```python
from build123d import *

# Parameters (mm, degrees)
F0_R     = 40.5
F1_DEPTH = 165
F2_W     = 77
F2_H     = 150
F3_DEPTH = 50.000001
F4_T     = -1.5
F5_R     = 40
F6_DEPTH = 165


with BuildPart() as f1:
    # F0 (on Top) → F1 (new body)
    with BuildSketch(Plane.XY):
        Circle(F0_R)
    extrude(amount=F1_DEPTH)

    # F2 (on Front) → F3 (cut)
    with BuildSketch(Plane.XZ):
        with Locations((0, 83.080945)):
            Rectangle(F2_W, F2_H)
    extrude(amount=F3_DEPTH, mode=Mode.SUBTRACT)

    # F4
    f4_openings = [f1.faces().sort_by_distance(p)[0] for p in [
        (0, 0, 165),
    ]]
    offset(amount=F4_T, openings=f4_openings)

    # F5 (on Top) → F6 (cut)
    with BuildSketch(Plane.XY):
        Circle(F5_R)
    extrude(amount=F6_DEPTH, mode=Mode.SUBTRACT)


solid = f1.part
```
Geometry check sheet. Reference: the model listing, model coordinates, mm. Coordinates: 2 decimals unless noted, no trailing zeros. Loops run counter-clockwise (first coordinate to the right, second up) from the corner with the lowest first, then second, coordinate; pieces in that order, holes last.
Item 1: Go/stop test with flat-tipped pins: pin 1 Ø6 at (x, z) = (-14, 104) entering from +Y; pin 2 Ø8 at (y, z) = (19, 128.5) entering from -X; pin 3 Ø9 at (x, y) = (-2.5, -32) entering from -Z; pin 4 Ø1 at (y, z) = (7.5, 21) entering from +X. Record where each tip stops, or that it passes through.
Item 2: Sectioned sample at D-D, the plane x = 25. Record the boundary of the cut face in (y, z), then the cut area to 3 significant figures.
Item 3: Sectioned sample at B-B, the plane x = 0. Record the boundary of the cut face in (y, z).
Item 4: Release check for a two-part mould opening along Z. For faces 1 (the face through (5.5, -39.9, 158.081)), 2 (the face through (-9.2, 39.2, 165)), 3 (the face through (-9.2, 39.2, 0)) record: released by +Z, released by -Z, zero draft, split by the parting line, or undercut.
Item 5: Sectioned sample at C-C, the plane y = -15.5. Record the boundary of the cut face in (x, z).
Item 6: Sectioned sample at A-A, the plane y = 0. Record the boundary of the cut face in (x, z), then the cut area to 3 significant figures.
Item 7: Thickness scan on line 1 (X direction, y = -1.5, z = 112.5); line 2 (Y direction, x = 0, z = 59); line 3 (X direction, y = 8, z = 87). Record the ranges inside material, lowest first.
Check result:
1. pin 1: stops at y = 38.98
1. pin 2: stops at x = -37.62
1. pin 3: passes through
1. pin 4: stops at x = 39.89
2. outline: (-31.86, 0) - (-31.22, 0) - (-31.22, 8.08) - (-31.86, 8.08) - close; (-31.86, 158.08) - (-31.22, 158.08) - (-31.22, 165) - (-31.86, 165) - close; (31.22, 0) - (31.86, 0) - (31.86, 165) - (31.22, 165) - close
2. area: 115 mm2
3. outline: (-40.5, 0) - (-40, 0) - (-40, 8.08) - (-40.5, 8.08) - close; (-40.5, 158.08) - (-40, 158.08) - (-40, 165) - (-40.5, 165) - close; (40, 0) - (40.5, 0) - (40.5, 165) - (40, 165) - close
4. face 1: undercut
4. face 2: released by +Z
4. face 3: released by -Z
5. outline: (-37.42, 0) - (-36.87, 0) - (-36.87, 8.08) - (-37.42, 8.08) - close; (-37.42, 158.08) - (-36.87, 158.08) - (-36.87, 165) - (-37.42, 165) - close; (36.87, 0) - (37.42, 0) - (37.42, 8.08) - (36.87, 8.08) - close; (36.87, 158.08) - (37.42, 158.08) - (37.42, 165) - (36.87, 165) - close
6. outline: (-40.5, 0) - (-40, 0) - (-40, 165) - (-40.5, 165) - close; (40, 0) - (40.5, 0) - (40.5, 165) - (40, 165) - close
6. area: 165 mm2
7. line 1: x = -40.47 to -39.97, 39.97 to 40.47
7. line 2: y = 40 to 40.5
7. line 3: x = -39.7 to -39.19, 39.19 to 39.7
